```python
from build123d import *

# Parameters (mm, degrees)
F0_W           = 23
F0_H           = 2
F1_DEPTH       = 23
F3_D           = 1
F3_DEPTH       = 3
F3_CBORE_D     = 19.5
F3_CBORE_DEPTH = 3
F3_TIP         = 0.3004303095
F4_R           = 11
F5_T1_DEPTH    = 80.1913118923
F6_T4_DEPTH    = 38.5721694425
F6_S5_R        = 12
F6_T6_DEPTH    = 21


# Not quite as in the source:
# - a fillet or chamfer that OpenCascade refuses, or shapes differently, is made with other operations: its cross-section is extruded or revolved along the edge and cut away or added


with BuildPart() as f1:
    # F0 (on Top) → F1 (new body)
    with BuildSketch(Plane.XY):
        with BuildLine():
            Line((-8.3816226795, 2), (-8.3816226795, 0))
            Line((-8.3816226795, 0), (14.6183773205, 0))
            ThreePointArc((14.6183773205, 0), (24.6183773205, -10), (14.6183773205, -20))
            Line((14.6183773205, -20), (-8.3816226795, -20))
            Line((-8.3816226795, -20), (-8.3816226795, -22))
            Line((-8.3816226795, -22), (14.6183773205, -22))
            ThreePointArc((14.6183773205, -22), (26.6183773205, -10), (14.6183773205, 2))
            Line((14.6183773205, 2), (-8.3816226795, 2))
        make_face()
        with Locations((3.1183773205, 3)):
            Rectangle(F0_W, F0_H)
    extrude(amount=F1_DEPTH)

    # F3
    with Locations(Plane(origin=(0, 4, 0), x_dir=(-1, 0, 0), z_dir=(0, 1, 0))):
        with Locations((-3.1183773205, 11.5)):
            CounterBoreHole(F3_D / 2, F3_CBORE_D / 2, F3_CBORE_DEPTH, depth=F3_DEPTH)
            with Locations((0, 0, -(F3_DEPTH + F3_TIP / 2))):  # 118° drill point
                Cone(0, F3_D / 2, F3_TIP, mode=Mode.SUBTRACT)

    # F4
    f4_edges = [f1.edges().sort_by_distance(p)[0] for p in [
        (-8.381623, 2, 23),
        (-8.381623, 2, 0),
        (-8.381623, -21, 0),
        (-8.381623, -21, 23),
    ]]
    fillet(f4_edges, radius=F4_R)

    # F5: chamfer of 11 x 1 on 1 edges, made by hand

    # F5_s2 → F5_t1 (cut)
    with BuildSketch(Plane.XY.offset(-28.5956559462)):
        Polygon((3.6183773205, 4), (14.6183773205, 3), (14.6183773205, 4), align=None)
    extrude(amount=F5_T1_DEPTH, mode=Mode.SUBTRACT)

    # F6: chamfer of 1 x 3 on 1 edges, made by hand


with BuildPart() as f6_tool2:
    # F6_s3 → F6_t4 (new body)
    with BuildSketch(Plane.XY.offset(-7.7860847213)):
        Polygon((11.6306977011, 3.2716072381), (14.6183773205, 2), (14.6183773205, 3), align=None)
    extrude(amount=F6_T4_DEPTH)

    # F6_s5 → F6_t6 (cut, symmetric)
    with BuildSketch(Plane.XY.offset(11.5)):
        with Locations((14.6183773205, -10)):
            Circle(F6_S5_R)
    extrude(amount=F6_T6_DEPTH, both=True, mode=Mode.SUBTRACT)


with BuildPart() as f1_1:
    add(f1.part)

    # F6_t1: cut F6_tool2
    add(f6_tool2.part, mode=Mode.SUBTRACT)


solid = f1_1.part
```
CAD build for the part. Positions are in the model's coordinates, mm. A direction names the side the tool comes from. Give positions to 0.01 mm unless a question says otherwise; leave off trailing zeros. Order: outer loops, then holes, each group sorted by start corner. A loop starts at its lowest first (then second) coordinate and runs counter-clockwise, first axis right, second up. Notation, with made-up numbers: M -36,13.5 L 2,13.5 A19 ccw 2,47.5 Z; hole C 47.25,32.25 d7. An arc over 180 degrees is marked long. Put each result on its own line as item: value. Start each with the question number.
(1) Saw through at B-B, the plane z = 12.75. Write the cut outline in (x, y), then the cut area to 3 significant figures.
(2) Flat gauge pins, fed straight in: pin 1 Ø1.5 at (y, z) = (-15, 15) entering from +X; pin 2 Ø4 at (y, z) = (-10, 7) entering from -X; pin 3 Ø4 at (x, z) = (6.5, 16.5) entering from +Y; pin 4 Ø10 at (x, y) = (-0.5, -13) entering from -Z. Where does each tip first touch, or does it go through?
(3) Drill centre lines: line 1 along Y through (x, z) = (4, 8.25); line 2 along X through (y, z) = (3.1, 11.5); line 3 along Y through (x, z) = (10.5, 21.5). Where is each one in solid material? Low to high.
(4) Saw through at A-A, the plane x = 21.5. Write the cut outline in (y, z).
(5) Saw through at D-D, the plane y = -10. Write the cut outline in (x, z).
(6) Mould opens along X. For faces 3 (the flat face through (3, 0, 11)), 4 (the cylindrical face through (24.616, -9.78, 11.339)), 5 (the cylindrical face through (-6.18, 2.52, 14.43)) say: +X half, -X half, draft (parallel to the pull), parting line (faces both ways), or undercut.
(7) Saw through at C-C, the plane x = 16. Write the cut outline in (y, z), then the cut area to 3 significant figures.
(8) Which spindle directions (+Z, -Z, +X, -X, +Y, -Y) get a long thin tool onto all of the face, cutting with end or side? Do faces 1 (the cylindrical face through (-5.245, 1.972, 3.308)), 2 (the flat face through (3, 1, 9)). Say none if no direction does.
Check result:
1. outline: M -8.36,-22 L 14.62,-22 A12 ccw 14.62,2 L 12.79,2.78 L 12.79,1 L -6.55,1 L -6.55,4 L -8.36,4 L -8.36,0 L 14.62,0 A10 cw 14.62,-20 L -8.36,-20 Z
1. area: 146 mm2
2. pin 1: stops at x = 25.84
2. pin 2: stops at x = 24.42
2. pin 3: stops at y = 1
2. pin 4: passes through
3. line 1: y = -22 to -20, 0 to 1
3. line 2: x = -8.38 to -6.63
3. line 3: y = -22 to -20, 0 to 3.37
4. outline: M -19.83,0 L -17.26,0 L -17.26,23 L -19.83,23 Z; M -2.74,0 L -0.17,0 L -0.17,23 L -2.74,23 Z
5. outline: M 24.62,0 L 26.62,0 L 26.62,23 L 24.62,23 Z
6. face 3: draft
6. face 4: -X half
6. face 5: undercut
7. outline: M -21.92,0 L -19.9,0 L -19.9,23 L -21.92,23 Z; M -0.1,0 L 1.92,0 L 1.92,23 L -0.1,23 Z
7. area: 92.7 mm2
8. face 1: -Z, -X, +Y, -Y
8. face 2: +Y
